Could you check a few things on this model? Use its own coordinates, in mm. A direction names the side the tool comes from. Give positions to 0.01 mm unless a question says otherwise; leave off trailing zeros. Order: outer loops, then holes, each group sorted by start corner. A loop starts at its lowest first (then second) coordinate and runs counter-clockwise, first axis right, second up. Notation, with made-up numbers: M 59,45 L 111,45 A24 ccw 111,84 Z; hole C 39.25,-9.5 d10. An arc over 180 degrees is marked long. Answer in a Markdown table with one row per item. Add a question column.
```python
from build123d import *

# Parameters (mm, degrees)
SM_BASE_FLANGE_1_DEPTH = 4
SKETCH_6_R             = 10
SKETCH_6_R_2           = 2.5
CUT_EXTRUDE_1_DEPTH    = 10
SKETCH_7_R             = 2
CUT_EXTRUDE_2_DEPTH    = 10
CUT_EXTRUDE_3_DEPTH    = 10
SKETCH_9_R             = 2
CUT_EXTRUDE_4_DEPTH    = 80
FILLET_2_R             = 2
SKETCH_10_R            = 1.5
CUT_EXTRUDE_5_DEPTH    = 4


# Sheet-metal steps are written as plain solids
with BuildPart() as part:
    # Sketch 1 → 基体-法兰1 (new body)
    with BuildSketch(Plane.XY):
        with BuildLine():
            Line((12.571428571, 79.00607055), (353.928571429, 24.689397047))
            ThreePointArc((353.928571429, 24.689397047), (375, 0), (353.928571429, -24.689397047))
            Line((353.928571429, -24.689397047), (12.571428571, -79.00607055))
            ThreePointArc((12.571428571, -79.00607055), (-80, 0), (12.571428571, 79.00607055))
        make_face()
    extrude(amount=-SM_BASE_FLANGE_1_DEPTH)

    # 草图6 → 切除-拉伸1 (cut)
    with BuildSketch(Plane.XY):
        Circle(SKETCH_6_R)
        with Locations((350, 0)):
            Circle(SKETCH_6_R_2)
    extrude(amount=-CUT_EXTRUDE_1_DEPTH, mode=Mode.SUBTRACT)

    # 草图7 → 切除-拉伸2 (cut)
    with BuildSketch(Plane.XY):
        with Locations((365, 0)):
            Circle(SKETCH_7_R)
        with Locations((350, -15)):
            Circle(SKETCH_7_R)
        with Locations((335, 0)):
            Circle(SKETCH_7_R)
        with Locations((350, 15)):
            Circle(SKETCH_7_R)
        with BuildLine():
            Line((111.294862901, 32.919806827), (111.294862901, -32.919806827))
            Line((111.294862901, -32.919806827), (56.389238276, -41.656377743))
            ThreePointArc((56.389238276, -41.656377743), (53.378656764, -40.291367953), (53.450847511, -36.986577299))
            ThreePointArc((53.450847511, -36.986577299), (62.032293151, -19.416348946), (64.999939097, -0.088979461))
            ThreePointArc((64.999939097, -0.088979461), (62.058814357, 19.33141383), (53.450847511, 36.986577299))
            ThreePointArc((53.450847511, 36.986577299), (53.378656764, 40.291367953), (56.389238276, 41.656377743))
            Line((56.389238276, 41.656377743), (111.294862901, 32.919806827))
        make_face()
        Polygon((141.940088648, 28.043545246), (141.940088648, -28.043545246), (318.181818182, 0), align=None)
        with BuildLine():
            ThreePointArc((0, 39), (-10.093942759, 37.671107225), (-19.5, 33.774990748))
            ThreePointArc((-19.5, 33.774990748), (-20.964101615, 28.310889132), (-15.5, 26.846787517))
            ThreePointArc((-15.5, 26.846787517), (-8.023390398, 29.943700615), (0, 31))
            ThreePointArc((0, 31), (4, 35), (0, 39))
        make_face()
        with BuildLine():
            ThreePointArc((26.846787517, 15.5), (21.920310217, 21.920310217), (15.5, 26.846787517))
            ThreePointArc((15.5, 26.846787517), (14.035898385, 32.310889132), (19.5, 33.774990748))
            ThreePointArc((19.5, 33.774990748), (27.577164466, 27.577164466), (33.774990748, 19.5))
            ThreePointArc((33.774990748, 19.5), (32.310889132, 14.035898385), (26.846787517, 15.5))
        make_face()
        with BuildLine():
            ThreePointArc((26.846787517, -15.5), (29.943700615, -8.023390398), (31, 0))
            ThreePointArc((31, 0), (35, 4), (39, 0))
            ThreePointArc((39, 0), (37.671107225, -10.093942759), (33.774990748, -19.5))
            ThreePointArc((33.774990748, -19.5), (28.310889132, -20.964101615), (26.846787517, -15.5))
        make_face()
        with BuildLine():
            ThreePointArc((0, -31), (8.023390398, -29.943700615), (15.5, -26.846787517))
            ThreePointArc((15.5, -26.846787517), (20.964101615, -28.310889132), (19.5, -33.774990748))
            ThreePointArc((19.5, -33.774990748), (10.093942759, -37.671107225), (0, -39))
            ThreePointArc((0, -39), (-4, -35), (0, -31))
        make_face()
        with BuildLine():
            ThreePointArc((-26.846787517, -15.5), (-21.920310217, -21.920310217), (-15.5, -26.846787517))
            ThreePointArc((-15.5, -26.846787517), (-14.035898385, -32.310889132), (-19.5, -33.774990748))
            ThreePointArc((-19.5, -33.774990748), (-27.577164466, -27.577164466), (-33.774990748, -19.5))
            ThreePointArc((-33.774990748, -19.5), (-32.310889132, -14.035898385), (-26.846787517, -15.5))
        make_face()
        with BuildLine():
            ThreePointArc((-26.846787517, 15.5), (-29.943700615, 8.023390398), (-31, 0))
            ThreePointArc((-31, 0), (-35, -4), (-39, 0))
            ThreePointArc((-39, 0), (-37.671107225, 10.093942759), (-33.774990748, 19.5))
            ThreePointArc((-33.774990748, 19.5), (-28.310889132, 20.964101615), (-26.846787517, 15.5))
        make_face()
    extrude(amount=-CUT_EXTRUDE_2_DEPTH, mode=Mode.SUBTRACT)

    # 草图8 → 切除-拉伸3 (cut)
    with BuildSketch(Plane.XY):
        with BuildLine():
            Line((347.5, 0), (337, 0))
            ThreePointArc((337, 0), (336.414213562, -1.414213562), (335, -2))
            Line((335, -2), (348.5, -2))
            ThreePointArc((348.5, -2), (347.763932023, -1.118033989), (347.5, 0))
        make_face()
        with BuildLine():
            ThreePointArc((335, 2), (336.414213562, 1.414213562), (337, 0))
            Line((337, 0), (347.5, 0))
            ThreePointArc((347.5, 0), (347.763932023, 1.118033989), (348.5, 2))
            Line((348.5, 2), (335, 2))
        make_face()
        with BuildLine():
            ThreePointArc((351.5, 2), (352.236067977, 1.118033989), (352.5, 0))
            Line((352.5, 0), (363, 0))
            ThreePointArc((363, 0), (363.585786438, 1.414213562), (365, 2))
            Line((365, 2), (351.5, 2))
        make_face()
        with BuildLine():
            Line((363, 0), (352.5, 0))
            ThreePointArc((352.5, 0), (352.236067977, -1.118033989), (351.5, -2))
            Line((351.5, -2), (365, -2))
            ThreePointArc((365, -2), (363.585786438, -1.414213562), (363, 0))
        make_face()
    extrude(amount=-CUT_EXTRUDE_3_DEPTH, mode=Mode.SUBTRACT)

    # 草图9 → 切除-拉伸4 (cut)
    with BuildSketch(Plane.XY):
        with Locations((120, 41.660451514)):
            Circle(SKETCH_9_R)
        with Locations((120, -41.660451514)):
            Circle(SKETCH_9_R)
    extrude(amount=-CUT_EXTRUDE_4_DEPTH, mode=Mode.SUBTRACT)

    # 圆角2
    fillet_2_edges = [part.edges().sort_by_distance(p)[0] for p in [
        (111.294862901, 32.919806827, -2),
        (111.294862901, -32.919806827, -2),
        (141.940088648, 28.043545246, -2),
        (318.181818182, 0, -2),
        (141.940088648, -28.043545246, -2),
    ]]
    fillet(fillet_2_edges, radius=FILLET_2_R)

    # 草图10 → 切除-拉伸5 (cut)
    with BuildSketch(Plane.XY):
        with Locations((0, 15)):
            Circle(SKETCH_10_R)
        with Locations((12.990381057, 7.5)):
            Circle(SKETCH_10_R)
        with Locations((12.990381057, -7.5)):
            Circle(SKETCH_10_R)
        with Locations((0, -15)):
            Circle(SKETCH_10_R)
        with Locations((-12.990381057, -7.5)):
            Circle(SKETCH_10_R)
        with Locations((-12.990381057, 7.5)):
            Circle(SKETCH_10_R)
    extrude(amount=-CUT_EXTRUDE_5_DEPTH, mode=Mode.SUBTRACT)


solid = part.part
```
1. Thinking about a two-plate mould opening in X: for faces 1 (the flat face through (226.142, 14.645, -1.972)), 2 (the flat face through (100, 37, 0)), 3 (the flat face through (180.86, 52.23, -1.97)), which applies, pulls with the +X half, pulls with the -X half, needs draft (parallel to the pull), parting line crosses it, or undercut?
2. If I drill on line 1 along Y through (x, z) = (12, -2.95); line 2 along Y through (x, z) = (347, -1.5); line 3 along Y through (x, z) = (68.5, -2.35), over which ranges is the centre line in solid material (lowest first)? Write a range as [from, to].
3. For faces 4 (the flat face through (100, 37, -4)), 5 (the cylindrical face through (-22, -21.84, -1.97)), which set-ups out of +Z, -Z, +X, -X, +Y, -Y let a thin tool reach every point of the face, with its end or its side?
4. Suppose I cut it at A-A on x = 343.5. List the corners of the cut face in (y, z) for me, plus the area to 3 significant figures.
5. Suppose I cut it at B-B on x = 218. List the corners of the cut face in (y, z) for me.
6. Suppose I cut it at C-C on y = -65. List the corners of the cut face in (x, z) for me.
7. Suppose I cut it at D-D on z = -2.6. Count the separate pieces of the cut face and the enclosed holes in it, plus the area to 3 significant figures.
8. Will these pins go through, and if not, where does the flat tip stop? P1, Ø1.5, axis at y = 51.5, z = -1, coming from the -X side; P2, Ø2, axis at y = 22.5, z = -3.5, coming from the +X side; P3, Ø1.8, axis at x = 0, y = 15, coming from the +Z side; P4, Ø2, axis at x = 343.5, z = -1.5, coming from the -Y side.
Findings below:
| question | item | result |
|---|---|---|
| 1 | face 1 | undercut |
| 1 | face 2 | needs draft |
| 1 | face 3 | pulls with the +X half |
| 2 | line 1 | [-79.09, -37.11], [-28.58, -8.63], [-6.37, 6.37], [8.63, 79.09] |
| 2 | line 2 | [-25.79, -2], [2, 25.79] |
| 2 | line 3 | [-70.11, -39.73], [39.73, 70.11] |
| 3 | face 4 | -Z, +X, -X, +Y, -Y |
| 3 | face 5 | +Z, -Z |
| 4 | outline | M -26.35,-4 L -2,-4 L -2,0 L -26.35,0 Z; M 2,-4 L 26.35,-4 L 26.35,0 L 2,0 Z |
| 4 | area | 195 mm2 |
| 5 | outline | M -46.32,-4 L -15.94,-4 L -15.94,0 L -46.32,0 Z; M 15.94,-4 L 46.32,-4 L 46.32,0 L 15.94,0 Z |
| 6 | outline | M -46.64,-4 L 100.59,-4 L 100.59,0 L -46.64,0 Z |
| 7 | separate pieces | 1 |
| 7 | enclosed holes | 20 |
| 7 | area | 37,800 mm2 |
| 8 | P1 | x = -61.84 |
| 8 | P2 | x = 362.76 |
| 8 | P3 | through |
| 8 | P4 | y = -26.51 |
